Verification items for the finished model (mm, model axes). Coordinates: 2 decimals unless noted, no trailing zeros. Write each loop counter-clockwise with the first axis right and the second up, starting at its lowest first coordinate (ties: lowest second). Pieces come first, ordered by that corner, then holes. Notation, with made-up numbers: M 52,41 L 66,41 A33 cw 66,75 Z; hole C 5.25,45.25 d1. An arc over 180 degrees is marked long. One line per item, written item: value.
Autodesk Inventor part; units mm, degrees
ref_plane "YZ Plane" through (0, 0, 0) normal (1, 0, 0) x (0, 1, 0)
ref_plane "XZ Plane" through (0, 0, 0) normal (0, 1, 0) x (-1, 0, 0)
ref_plane "XY Plane" through (0, 0, 0) normal (0, 0, 1) x (1, 0, 0)
sketch "Sketch1" plane through (0, 0, 0) normal (0, 0, 1) x (1, 0, 0)
  line L0 (-77.5, 17.5) -> (77.5, 17.5)
  line L1 (77.5, 17.5) -> (77.5, -17.5)
  line L2 (77.5, -17.5) -> (-77.5, -17.5)
  line L3 (-77.5, -17.5) -> (-77.5, 17.5)
  point P0 (0, 0)
  point P1 (0, 17.5)
  point P2 (-77.5, 0)
  dimension "d0" = 155
  dimension "d1" = 35
extrude "Extrusion1" add sketch "Sketch1" along normal blind 8
sketch "Sketch4" plane through (0, 0, 8) normal (0, 0, 1) x (1, 0, 0)
  line L0 (-73.5, -11.5) -> (73.5, -11.5) construction
  line L1 (73.5, -11.5) -> (73.5, 11.5) construction
  line L2 (73.5, 11.5) -> (-73.5, 11.5) construction
  line L3 (-73.5, 11.5) -> (-73.5, -11.5) construction
  line L4 (-77.5, 17.5) -> (-77.5, -17.5) construction
  line L5 (77.5, 17.5) -> (-77.5, 17.5) construction
  point P0 (0, 0)
  point P1 (-73.5, 0)
  point P2 (-77.5, 0)
  point P3 (0, 11.5)
  point P4 (0, 17.5)
  dimension "d19" = 4
  dimension "d20" = 6
hole "Hole1" at (73.5, -11.5, 8) at (73.5, 11.5, 8) direction (0, 0, -1) diameter 4.5 end through all
sketch "Sketch5" plane through (0, 0, 8) normal (0, 0, 1) x (1, 0, 0)
  circle A0 centre (23.5, 3.5) radius 2.3
  circle A1 centre (23.5, 12.5) radius 1.5001
  point P0 (0, 0)
  point P1 (98.6998, 12.5)
hole "Hole2" at (98.6998, 12.5, 8) at (23.5, 3.5, 8) at (23.5, 12.5, 8) direction (0, 0, -1) diameter 4 end through all
properties part number "0005-10-008" material "Wood (Maple)"
Item 1: Cross-section at A-A, the plane y = -11.5. Enter the section's corners in (x, z).
The answers:
outline: M -77.5,0 L 71.25,0 L 71.25,8 L -77.5,8 Z; M 75.75,0 L 77.5,0 L 77.5,8 L 75.75,8 Z
Item 2: Scan lines: line 1 (Y direction, x = 73.5, z = 5); line 2 (Y direction, x = 23.5, z = 6); line 3 (X direction, y = 10, z = 2). Record each from-to range of solid material in increasing order.
The answers:
line 1: y = -17.5 to -13.75, -9.25 to 9.25, 13.75 to 17.5
line 2: y = -17.5 to 1.5, 5.5 to 10.5, 14.5 to 17.5
line 3: x = -77.5 to 71.82, 75.18 to 77.5
Item 3: Draft check along X on faces 1 (the face through (-77.5, 0, 4)), 2 (the face through (-1, 0, 8)), 3 (the face through (77.5, 0, 4)), 4 (the face through (22.148, 13.974, 3.944)). Enter one of: released by +X, released by -X, zero draft, split by the parting line, or undercut.
The answers:
face 1: released by -X
face 2: zero draft
face 3: released by +X
face 4: undercut
Item 4: Cross-section at B-B, the plane x = 23.5. Enter the section's corners in (y, z).
The answers:
outline: M -17.5,0 L 1.5,0 L 1.5,8 L -17.5,8 Z; M 5.5,0 L 10.5,0 L 10.5,8 L 5.5,8 Z; M 14.5,0 L 17.5,0 L 17.5,8 L 14.5,8 Z
Item 5: Cross-section at C-C, the plane y = 3.5. Enter the section's corners in (x, z), and give its area (3 significant figures).
The answers:
outline: M -77.5,0 L 21.5,0 L 21.5,8 L -77.5,8 Z; M 25.5,0 L 77.5,0 L 77.5,8 L 25.5,8 Z
area: 1,210 mm²
Item 6: Go/stop test with a flat-tipped pin: P1, Ø2.5, axis at x = 23.5, y = 12.5, coming from the -Z side. Record where the tip stops, or that it passes through.
The answers:
P1: passes through
